```python
from build123d import *

# Parameters (mm, degrees)
CHANFREIN1_SIZE         = 1
CHANFREIN2_SIZE         = 0.5
ENL_V_MAT_EXTRU_1_REACH = 106.47
ESQUISSE2_W             = 5.137351374
ESQUISSE2_H             = 15.268552686


with BuildPart() as part:
    # Esquisse1 → Révolution1 (revolve)
    with BuildSketch(Plane.XY, mode=Mode.PRIVATE) as r_volution1_sk:
        Polygon((0, 0), (0, 5), (12, 5), (12, 5.118365096), (17, 6), (31, 6), (31, 5.8), (32.5, 5.8), (32.5, 6), (35, 6), (35, 5.4), (36.5, 5.4), (36.5, 6), (99, 6), (99, 4), (102, 4), (102, 7), (104, 7), (104, 0), (103.330760558, 0), align=None)
    revolve(r_volution1_sk.sketch.rotate(Axis((0, 0, 0), (1, 0, 0)), 90), axis=Axis((0, 0, 0), (1, 0, 0)))

    # Chanfrein1
    chanfrein1_edges = [part.edges().sort_by_distance(p)[0] for p in [
        (0, 0, -5),
    ]]
    chamfer(chanfrein1_edges, length=CHANFREIN1_SIZE)

    # Chanfrein2
    chanfrein2_edges = [part.edges().sort_by_distance(p)[0] for p in [
        (36.5, 0, -6),
    ]]
    chamfer(chanfrein2_edges, length=CHANFREIN2_SIZE)

    # Esquisse2 → Enlèv. mat.-Extru.1 (cut, up to next)
    with BuildSketch(Plane(origin=(104, 0, 0), x_dir=(0, 0, -1), z_dir=(1, 0, 0)), mode=Mode.PRIVATE) as enl_v_mat_extru_1_sk1:
        with Locations((-6.568675687, -0.086100861)):
            Rectangle(ESQUISSE2_W, ESQUISSE2_H)
    enl_v_mat_extru_1_tool1 = extrude(enl_v_mat_extru_1_sk1.sketch, amount=-ENL_V_MAT_EXTRU_1_REACH, mode=Mode.PRIVATE) & part.part
    # Esquisse2 → Enlèv. mat.-Extru.1 (cut, up to next)
    with BuildSketch(Plane(origin=(104, 0, 0), x_dir=(0, 0, -1), z_dir=(1, 0, 0)), mode=Mode.PRIVATE) as enl_v_mat_extru_1_sk2:
        with Locations((6.568675687, -0.086100861)):
            Rectangle(ESQUISSE2_W, ESQUISSE2_H)
    enl_v_mat_extru_1_tool2 = extrude(enl_v_mat_extru_1_sk2.sketch, amount=-ENL_V_MAT_EXTRU_1_REACH, mode=Mode.PRIVATE) & part.part
    add(enl_v_mat_extru_1_tool1.solids().sort_by_distance((104, -0.086101, 6.568676))[0], mode=Mode.SUBTRACT)
    add(enl_v_mat_extru_1_tool2.solids().sort_by_distance((104, -0.086101, -6.568676))[0], mode=Mode.SUBTRACT)


solid = part.part
```
Build history of the part. All positions in model axes, mm. A direction names the side the tool comes from. Round coordinates to 2 decimals unless told otherwise and drop trailing zeros. Order: outer loops, then holes, each group sorted by start corner. A loop starts at its lowest first (then second) coordinate and runs counter-clockwise, first axis right, second up. Notation, with made-up numbers: (80.5, 51) -> (95.5, 51) arc R16 cw to (95.5, 78) -> close; hole circle Ø1 at (80.5, 37.25). An arc over 180 degrees is marked (long way). Answer in a Markdown table with one row per item.
1) Band-saw the part on B-B on x = 76.5. Give the cut face in (y, z), and give its area (3 significant figures).
Values:
| item | result |
|---|---|
| outline | circle Ø12 at (0, 0) |
| area | 113 mm2 |
2) Wall check: L1, parallel to X at y = -4.75, z = -1.75; L2, parallel to Z at x = 52, y = -1.75; L3, parallel to X at y = -3.5, z = -2. Give the ranges that are in metal, low to high.
Values:
| item | result |
|---|---|
| L1 | 12 to 99, 102 to 104 |
| L2 | -5.74 to 5.74 |
| L3 | 0.03 to 99, 102 to 104 |
3) Pin check, flat tips, straight feed: P1, Ø0.6, axis at x = 102.5, y = 3, coming from the -Z side; P2, Ø0.6, axis at x = 103, y = 2.5, coming from the +Z side; P3, Ø2, axis at x = 50, z = 3.5, coming from the +Y side. Stop position of each tip, or through.
Values:
| item | result |
|---|---|
| P1 | z = -4 |
| P2 | z = 4 |
| P3 | y = 5.45 |
4) Which spindle directions (+Z, -Z, +X, -X, +Y, -Y) get a long thin tool onto all of the face, cutting with end or side? Do faces 4 (the cylindrical face through (35.76, 3.286, -4.285)), 5 (the cylindrical face through (33.768, -1.802, 5.723)), 6 (the cylindrical face through (103, 7, 0)). Say none if no direction does.
Values:
| item | result |
|---|---|
| face 4 | none |
| face 5 | -X |
| face 6 | +X, -X, +Y |
5) Mould opens along X. For faces 1 (the flat face through (104, 0, 0)), 2 (the flat face through (103, 0, 4)), 3 (the flat face through (102, 5, 0)) say: released by +X, released by -X, zero draft, split by the parting line, or undercut.
Values:
| item | result |
|---|---|
| face 1 | released by +X |
| face 2 | zero draft |
| face 3 | undercut |
6) Band-saw the part on A-A on x = 7.5. Give the cut face in (y, z), and give its area (3 significant figures).
Values:
| item | result |
|---|---|
| outline | circle Ø10 at (0, 0) |
| area | 78.5 mm2 |
